The listing builds one solid part. Answer for the finished solid, in the listing's coordinates (mm). A direction names the side the tool comes from. Round coordinates to 2 decimals unless told otherwise and drop trailing zeros. Write each loop counter-clockwise with the first axis right and the second up, starting at its lowest first coordinate (ties: lowest second). Pieces come first, ordered by that corner, then holes.
Item 1: Find section A-A on z = 6.5. Give the vertices of the cut face in (x, y).
Item 2: Find section C-C on y = -0.5. Give the vertices of the cut face in (x, z), then the cut area to 3 significant figures.
Item 3: Each of these flat-tipped pins is pushed along its axis until it touches: pin 1 (1 mm diameter, centred on x = 1.5, z = 2, fed in from -Y); pin 2 (2 mm diameter, centred on y = 1.5, z = 3.5, fed in from +X). Where does it stop, or does it pass through?
Item 4: Find section D-D on z = 3. Give the vertices of the cut face in (x, y).
Item 5: Find section B-B on x = 0. Give the vertices of the cut face in (y, z), then the cut area to 3 significant figures.
Item 6: Find the intervals of material crossed by probe 1 along Y at (x, z) = (0, 6.35); probe 2 along Z at (x, y) = (0.7, 1.75); probe 3 along Y at (x, z) = (-1.1, 6.75), in increasing order.
Item 7: A tool of negligible diameter and unlimited length cuts with its end or side. For faces 5 (the face through (-1.724, 1.014, 6.465)), 6 (the face through (2, 0, 4)), from which of +Z, -Z, +X, -X, +Y, -Y can it reach the whole face along a straight path? Write none if from no direction.
Item 8: For a pull along X with two mould halves and no side action, classify faces 1 (the face through (0, 0, 5)), 2 (the face through (-1.74, -0.99, 6.46)), 3 (the face through (0, 0, 0)), 4 (the face through (-1.5, 0.07, 7.03)) as +X half, -X half, draft (parallel to the pull), parting line (faces both ways), or undercut.
Autodesk Inventor part; units mm, degrees
ref_plane "YZ Plane" through (0, 0, 0) normal (1, 0, 0) x (0, 1, 0)
ref_plane "XZ Plane" through (0, 0, 0) normal (0, 1, 0) x (-1, 0, 0)
ref_plane "XY Plane" through (0, 0, 0) normal (0, 0, 1) x (1, 0, 0)
sketch "Sketch1" plane through (0, 0, 0) normal (0, 0, 1) x (1, 0, 0)
  circle A0 centre (0, 0) radius 1.5
  dimension "d0" = 3
extrude "Extrusion1" add sketch "Sketch1" along normal blind 4
sketch "Sketch2" plane through (0, 0, 4) normal (0, 0, 1) x (1, 0, 0)
  circle A0 centre (0, 0) radius 1.5 construction
  line L0 (0.866, 1.5) -> (1.7321, 0) construction
  line L1 (1.7321, 0) -> (0.866, -1.5)
  line L2 (0.866, -1.5) -> (-0.866, -1.5)
  line L3 (-0.866, -1.5) -> (-1.7321, 0)
  line L4 (-1.7321, 0) -> (-0.866, 1.5)
  line L5 (-0.866, 1.5) -> (0.866, 1.5)
  line L6 (2.3094, 0) -> (1.1547, 2)
  line L7 (1.1547, 2) -> (-1.1547, 2)
  line L8 (-1.1547, 2) -> (-2.3094, 0)
  line L9 (-2.3094, 0) -> (-1.1547, -2)
  line L10 (-1.1547, -2) -> (1.1547, -2)
  line L11 (1.1547, -2) -> (2.3094, 0)
  point P0 (0, 1.5)
  dimension "d3" = 0.5
extrude "Extrusion2" add sketch "Sketch2" along normal blind 5
sketch "Sketch3" plane through (0, 0, 9) normal (0, 0, 1) x (1, 0, 0)
  circle A0 centre (0, 0) radius 1.5
  dimension "d6" = 3
extrude "Extrusion3" cut sketch "Sketch3" against normal blind 4
properties part number "piedino"
Check values:
1. outline: (-2.31, 0) - (-1.15, -2) - (1.15, -2) - (2.31, 0) - (1.15, 2) - (-1.15, 2) - close; hole circle Ø3 at (0, 0)
2. outline: (-2.02, 4) - (-1.41, 4) - (-1.41, 0) - (1.41, 0) - (1.41, 4) - (2.02, 4) - (2.02, 9) - (1.41, 9) - (1.41, 5) - (-1.41, 5) - (-1.41, 9) - (-2.02, 9) - close
2. area: 20.2 mm2
3. pin 1: stops at y = -1.12
3. pin 2: stops at x = 1.94
4. outline: circle Ø3 at (0, 0)
5. outline: (-2, 4) - (-1.5, 4) - (-1.5, 0) - (1.5, 0) - (1.5, 4) - (2, 4) - (2, 9) - (1.5, 9) - (1.5, 5) - (-1.5, 5) - (-1.5, 9) - (-2, 9) - close
5. area: 20.0 mm2
6. probe 1: y = -2 to -1.5, 1.5 to 2
6. probe 2: z = 4 to 9
6. probe 3: y = -2 to -1.02, 1.02 to 2
7. face 5: +Z, -Z, -X, +Y
7. face 6: -Z
8. face 1: undercut
8. face 2: -X half
8. face 3: draft
8. face 4: undercut
